Job drawing, mm, ordinate dimensions from the low corner. One solid piece. A direction names the side the tool comes from. Give positions to 0.01 mm unless a question says otherwise; leave off trailing zeros. Write each loop counter-clockwise with the first axis right and the second up, starting at its lowest first coordinate (ties: lowest second). Pieces come first, ordered by that corner, then holes. Notation, with made-up numbers: (19, 64.5) - (47, 64.5) arc R21 ccw to (47, 90.5) - close; hole circle Ø5 at (15, 33.5). An arc over 180 degrees is marked (long way). Answer in a Markdown table with one row per item. Add a question column.
1. Which spindle directions (+Z, -Z, +X, -X, +Y, -Y) get a long thin tool onto all of the face, cutting with end or side? Do the marked faces 4, 5, 6 and 7. Say none if no direction does.
2. Probe line 1 along Y through (x, z) = (70, 3.1); line 2 along Y through (x, z) = (37, 2.3). List the from-to ranges inside material, lowest first.
3. Band-saw the part on D-D on x = 57. Write the cut outline in (y, z), plus the area to 3 significant figures.
4. Band-saw the part on B-B on y = 68.5. Write the cut outline in (x, z), plus the area to 3 significant figures.
5. Pull direction X, two halves, no side cores. Call the marked faces 1, 2 and 3: released by +X, released by -X, zero draft, split by the parting line, or undercut.
6. Band-saw the part on A-A on x = 37. Write the cut outline in (y, z), plus the area to 4 significant figures.
7. Drop flat-ended pins along their axis: pin 1 Ø3 at (y, z) = (17.5, 2.5) entering from +X; pin 2 Ø1.5 at (x, z) = (63.5, 2) entering from +Y; pin 3 Ø1 at (x, z) = (36, 2.5) entering from -Y. Give the stop position or say it passes through.
8. Band-saw the part on C-C on y = 37. Write the cut outline in (x, z).
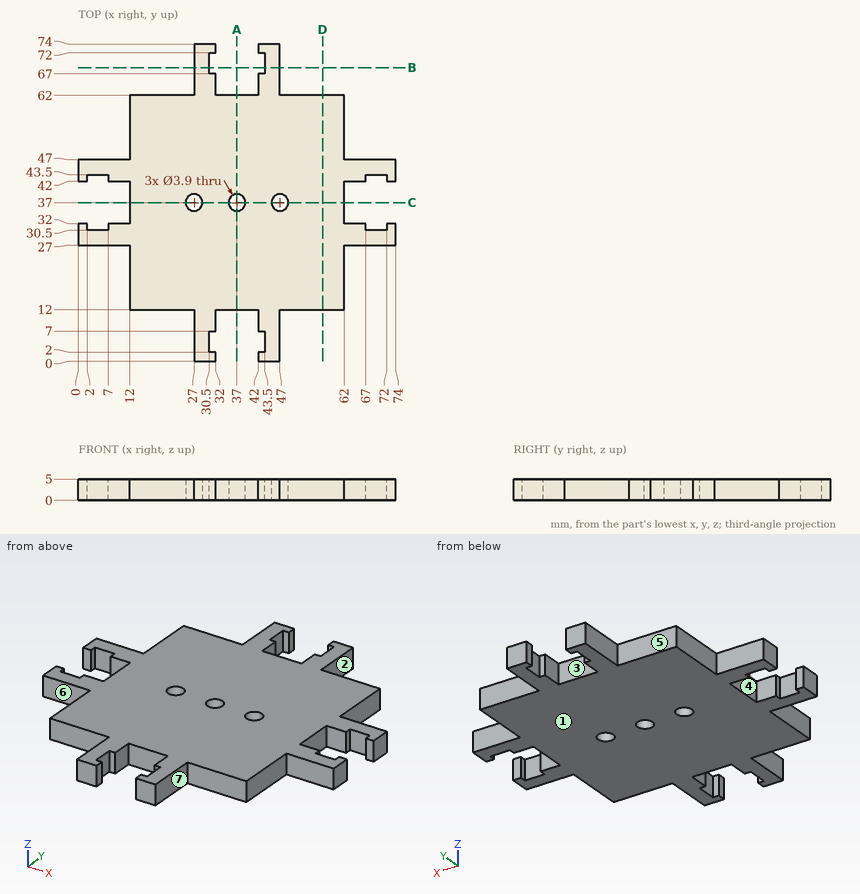
Values:
| question | item | result |
|---|---|---|
| 1 | face 4 | +Z, -Z, -X |
| 1 | face 5 | +Z, -Z, -X, +Y |
| 1 | face 6 | +Z, -Z, -X, -Y |
| 1 | face 7 | +Z, -Z, +X, -Y |
| 2 | line 1 | y = 27 to 30.5, 43.5 to 47 |
| 2 | line 2 | y = 12 to 35.05, 38.95 to 62 |
| 3 | outline | (12, 0) - (62, 0) - (62, 5) - (12, 5) - close |
| 3 | area | 250 mm² |
| 4 | outline | (27, 0) - (30.5, 0) - (30.5, 5) - (27, 5) - close; (43.5, 0) - (47, 0) - (47, 5) - (43.5, 5) - close |
| 4 | area | 35.0 mm² |
| 5 | face 1 | zero draft |
| 5 | face 2 | released by +X |
| 5 | face 3 | undercut |
| 6 | outline | (12, 0) - (35.05, 0) - (35.05, 5) - (12, 5) - close; (38.95, 0) - (62, 0) - (62, 5) - (38.95, 5) - close |
| 6 | area | 230.5 mm² |
| 7 | pin 1 | stops at x = 62 |
| 7 | pin 2 | stops at y = 47 |
| 7 | pin 3 | stops at y = 12 |
| 8 | outline | (12, 0) - (25.05, 0) - (25.05, 5) - (12, 5) - close; (28.95, 0) - (35.05, 0) - (35.05, 5) - (28.95, 5) - close; (38.95, 0) - (45.05, 0) - (45.05, 5) - (38.95, 5) - close; (48.95, 0) - (62, 0) - (62, 5) - (48.95, 5) - close |
